Geometry: final body of the model. Coordinates: model frame, mm. A direction names the side the tool comes from. Give positions to 0.01 mm unless a question says otherwise; leave off trailing zeros. Write each loop counter-clockwise with the first axis right and the second up, starting at its lowest first coordinate (ties: lowest second). Pieces come first, ordered by that corner, then holes.
Q1. Reachability of faces 1 (the face through (0, -97.942, 3)), 2 (the face through (0, -53.5, 13)) from +Z, -Z, +X, -X, +Y, -Y: full face, straight path, thin tool, end or side. Return the list, or none.
Q2. Cut plane A-A on y = -12. Return the cut outline in (x, z), plus the area to 3 significant figures.
Q3. Pin query (flat end, axial travel): pin 1 (1 mm diameter, centred on y = 35, z = 7, fed in from +X) (3 decimals); pin 2 (3 mm diameter, centred on x = -20, z = 3.5, fed in from -Y); pin 3 (1.5 mm diameter, centred on x = 17, z = 12.5, fed in from -Y). Return the tip coordinate at first contact, or that it passes through.
Q4. Cut plane B-B on z = 2. Return the cut outline in (x, y).
Q5. Line query: L1, parallel to X at y = -1, z = 11; L2, parallel to Z at x = -2, y = -73.5; L3, parallel to X at y = -14, z = 7.5. Output: solid intervals per line, ascending.
```python
from build123d import *

# Parameters (mm, degrees)
PAD_DEPTH    = 14
FILLET001_R  = 4
FILLET002_R  = 16
FILLET_R     = 7
SKETCH059_W  = 80
SKETCH059_H  = 50
POCKET_DEPTH = 3


with BuildPart() as part:
    # Sketch → Pad (new body)
    with BuildSketch(Plane.XY):
        with BuildLine():
            Line((-35, -53.5), (-35, -69.5))
            Line((-35, -69.5), (-4.5, -97.94171))
            Line((-4.5, -97.94171), (4.5, -97.94171))
            Line((4.5, -97.94171), (35, -69.5))
            Line((35, -69.5), (35, -53.5))
            Line((35, 33.5), (35, -53.5))
            ThreePointArc((35, 33.5), (29.142136, 47.642136), (15, 53.5))
            Line((-15, 53.5), (15, 53.5))
            ThreePointArc((-15, 53.5), (-29.142136, 47.642136), (-35, 33.5))
            Line((-35, 33.5), (-35, -53.5))
        make_face()
    extrude(amount=PAD_DEPTH)

    # Fillet001
    fillet001_edges = [part.edges().sort_by_distance(p)[0] for p in [
        (-4.5, -97.94171, 7),
        (4.5, -97.94171, 7),
    ]]
    fillet(fillet001_edges, radius=FILLET001_R)

    # Fillet002
    fillet002_edges = [part.edges().sort_by_distance(p)[0] for p in [
        (35, -69.5, 7),
        (-35, -69.5, 7),
    ]]
    fillet(fillet002_edges, radius=FILLET002_R)

    # Fillet
    fillet_edges = [part.edges().sort_by_distance(p)[0] for p in [
        (-17.782163, -85.555893, 14),
        (-33.672961, -68.922987, 14),
        (-4.390363, -97.66338, 14),
        (-35, -58.021501, 14),
        (0, -97.94171, 14),
        (-35, -10, 14),
        (4.390363, -97.66338, 14),
        (-29.142136, 47.642136, 14),
        (17.782163, -85.555893, 14),
        (0, 53.5, 14),
        (33.672961, -68.922987, 14),
        (29.142136, 47.642136, 14),
        (35, -58.021501, 14),
        (35, -10, 14),
    ]]
    fillet(fillet_edges, radius=FILLET_R)

    # Sketch059 (on Face8 of Clone015) → Pocket (cut)
    with BuildSketch(Plane.XY.offset(14)):
        with Locations((0, -78.5)):
            Rectangle(SKETCH059_W, SKETCH059_H)
    extrude(amount=-POCKET_DEPTH, mode=Mode.SUBTRACT)


solid = part.part
```
Data:
1. face 1: +Z, -Z, +X, -X, -Y
1. face 2: +Z, +X, -X, -Y
2. outline: (-35, 0) - (35, 0) - (35, 7) arc R7 ccw to (28, 14) - (-28, 14) arc R7 ccw to (-35, 7) - close
2. area: 959 mm2
3. pin 1: stops at x = 34.975
3. pin 2: stops at y = -84.89
3. pin 3: stops at y = -53.5
4. outline: (-35, -62.54) arc R16 ccw to (-29.91, -74.24) - (-5.65, -96.87) arc R4 ccw to (-2.92, -97.94) - (2.92, -97.94) arc R4 ccw to (5.65, -96.87) - (29.91, -74.24) arc R16 ccw to (35, -62.54) - (35, 33.5) arc R20 ccw to (15, 53.5) - (-15, 53.5) arc R20 ccw to (-35, 33.5) - close
5. L1: x = -33.74 to 33.74
5. L2: z = 0 to 11
5. L3: x = -34.98 to 34.98
